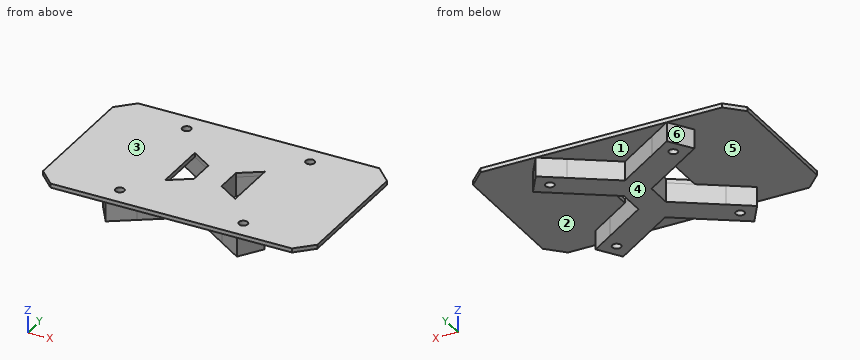
from build123d import *

# Parameters (mm, degrees)
SKETCH1_R           = 1.6
BOSS_EXTRUDE1_DEPTH = 7
SKETCH2_W           = 100
SKETCH2_H           = 58.867504906
SKETCH2_R           = 1.6
BOSS_EXTRUDE2_DEPTH = 1.5
CHAMFER1_SIZE       = 6
CHAMFER2_SIZE       = 6


with BuildPart() as part:
    # Sketch1 → Boss-Extrude1 (new body)
    with BuildSketch(Plane.XY):
        Polygon((-21.113249509, 15.566247547), (-5, 4.824081208), (-5, -4.824081208), (-21.113249509, -15.566247547), (-25.273500981, -18.339748528), (-29.433752453, -21.113249509), (-23.886750491, -29.433752453), (-19.726499019, -26.660251472), (-15.566247547, -23.886750491), (0, -13.509252126), (15.566247547, -23.886750491), (19.726499019, -26.660251472), (23.886750491, -29.433752453), (29.433752453, -21.113249509), (25.273500981, -18.339748528), (21.113249509, -15.566247547), (5, -4.824081208), (5, 4.824081208), (21.113249509, 15.566247547), (25.273500981, 18.339748528), (29.433752453, 21.113249509), (23.886750491, 29.433752453), (19.726499019, 26.660251472), (15.566247547, 23.886750491), (0, 13.509252126), (-15.566247547, 23.886750491), (-19.726499019, 26.660251472), (-23.886750491, 29.433752453), (-29.433752453, 21.113249509), (-25.273500981, 18.339748528), align=None)
        with Locations((-22.5, -22.5)):
            Circle(SKETCH1_R, mode=Mode.SUBTRACT)
        with Locations((22.5, -22.5)):
            Circle(SKETCH1_R, mode=Mode.SUBTRACT)
        with Locations((-22.5, 22.5)):
            Circle(SKETCH1_R, mode=Mode.SUBTRACT)
        with Locations((22.5, 22.5)):
            Circle(SKETCH1_R, mode=Mode.SUBTRACT)
    extrude(amount=BOSS_EXTRUDE1_DEPTH)

    # Sketch2 → Boss-Extrude2 (add)
    with BuildSketch(Plane.XY.offset(7)):
        Rectangle(SKETCH2_W, SKETCH2_H)
        Polygon((-12.763878189, -10), (-12.763878189, 10), (-5, 4.824081208), (-5, -4.824081208), align=None, mode=Mode.SUBTRACT)
        Polygon((12.763878189, 10), (12.763878189, -10), (5, -4.824081208), (5, 4.824081208), align=None, mode=Mode.SUBTRACT)
        with Locations((-22.5, 22.5)):
            Circle(SKETCH2_R, mode=Mode.SUBTRACT)
        with Locations((22.5, 22.5)):
            Circle(SKETCH2_R, mode=Mode.SUBTRACT)
        with Locations((22.5, -22.5)):
            Circle(SKETCH2_R, mode=Mode.SUBTRACT)
        with Locations((-22.5, -22.5)):
            Circle(SKETCH2_R, mode=Mode.SUBTRACT)
    extrude(amount=BOSS_EXTRUDE2_DEPTH)

    # Chamfer1
    chamfer1_edges = [part.edges().sort_by_distance(p)[0] for p in [
        (-50, -29.433752453, 7.75),
    ]]
    chamfer(chamfer1_edges, length=CHAMFER1_SIZE)

    # Chamfer2
    chamfer2_edges = [part.edges().sort_by_distance(p)[0] for p in [
        (50, 29.433752453, 7.75),
        (-50, 29.433752453, 7.75),
        (50, -29.433752453, 7.75),
    ]]
    chamfer(chamfer2_edges, length=CHAMFER2_SIZE)


solid = part.part
Design review of the part built by this model. Coordinates are the model's own, in mm. Face numbers are marked on the shaded views. A direction names the side the tool comes from. Round coordinates to 2 decimals unless told otherwise and drop trailing zeros. Order: outer loops, then holes, each group sorted by start corner. A loop starts at its lowest first (then second) coordinate and runs counter-clockwise, first axis right, second up.
1) Machinability: for the marked faces 1, 2 and 3, which of the approach directions +Z, -Z, +X, -X, +Y, -Y give a long, thin tool a straight path to every point of the face, cutting with its end or side? Answer none if there is none.
The answers:
face 1: -Z, +Y
face 2: -Z, +X
face 3: +Z, +X, -X, +Y, -Y
2) Consider section C-C (x = 22.5). State the section outline as (y, z) points, plus the area to 3 significant figures.
The answers:
outline: (-29.43, 7) - (-28.51, 7) - (-28.51, 0) - (-24.1, 0) - (-24.1, 8.5) - (-29.43, 8.5) - close; (-20.9, 0) - (-16.49, 0) - (-16.49, 7) - (16.49, 7) - (16.49, 0) - (20.9, 0) - (20.9, 8.5) - (-20.9, 8.5) - close; (24.1, 0) - (28.51, 0) - (28.51, 7) - (29.43, 7) - (29.43, 8.5) - (24.1, 8.5) - close
area: 202 mm2
3) Consider section D-D (x = -8). State the section outline as (y, z) points.
The answers:
outline: (-29.43, 7) - (-18.84, 7) - (-18.84, 0) - (-6.82, 0) - (-6.82, 8.5) - (-29.43, 8.5) - close; (6.82, 0) - (18.84, 0) - (18.84, 7) - (29.43, 7) - (29.43, 8.5) - (6.82, 8.5) - close
4) Clearance check with flat-ended pins moving along their axes: pin 1 Ø2.5 at (y, z) = (0, 5) entering from +X; pin 2 Ø1 at (x, z) = (24.5, 3) entering from +Y; pin 3 Ø3.5 at (x, y) = (22.5, -22.5) entering from +Z; pin 4 Ø1.5 at (y, z) = (-23, 1.5) entering from +X. State where each tip first meets the part, or that it passes through.
The answers:
pin 1: stops at x = 5
pin 2: stops at y = 29.26
pin 3: stops at z = 8.5
pin 4: stops at x = 28.68
5) Consider section A-A (z = 5). State the section outline as (x, y) points.
The answers:
outline: (-29.43, -21.11) - (-23.89, -29.43) - (0, -13.51) - (23.89, -29.43) - (29.43, -21.11) - (5, -4.82) - (5, 4.82) - (29.43, 21.11) - (23.89, 29.43) - (0, 13.51) - (-23.89, 29.43) - (-29.43, 21.11) - (-5, 4.82) - (-5, -4.82) - close; hole circle Ø3.2 at (-22.5, -22.5); hole circle Ø3.2 at (-22.5, 22.5); hole circle Ø3.2 at (22.5, -22.5); hole circle Ø3.2 at (22.5, 22.5)
6) Draft analysis for pull direction Y (two halves, no side actions). For the marked faces 4, 5 and 6, state which applies: released by +Y, released by -Y, zero draft, split by the parting line, or undercut.
The answers:
face 4: zero draft
face 5: undercut
face 6: released by +Y
7) Consider section B-B (y = -2.5). State the section outline as (x, z) points.
The answers:
outline: (-50, 7) - (-12.76, 7) - (-12.76, 8.5) - (-50, 8.5) - close; (-5, 0) - (5, 0) - (5, 8.5) - (-5, 8.5) - close; (12.76, 7) - (50, 7) - (50, 8.5) - (12.76, 8.5) - close
8) For L1, parallel to X at y = -2, z = 7.75; L2, parallel to Y at x = 22.5, z = 3.5; L3, parallel to Z at x = 42, y = -18, list the stretches that pass through material, from the lowest coordinate up.
The answers:
L1: x = -50 to -12.76, -5 to 5, 12.76 to 50
L2: y = -28.51 to -24.1, -20.9 to -16.49, 16.49 to 20.9, 24.1 to 28.51
L3: z = 7 to 8.5
